from build123d import *
from build123d.topology import SkipClean

# Parameters (mm, degrees)
SKETCH2_R           = 1.65
SKETCH2_R_2         = 11.25
BOSS_EXTRUDE2_DEPTH = 2.5
SKETCH7_W           = 42.3
SKETCH7_H           = 35
BOSS_EXTRUDE5_DEPTH = 2
BOSS_EXTRUDE6_DEPTH = 2.5
FILLET2_R           = 5
FILLET3_R           = 3
SKETCH11_R          = 1.65
CUT_EXTRUDE1_DEPTH  = 2
SKETCH12_W          = 42.3
SKETCH12_H          = 35
SKETCH12_R          = 1.65
BOSS_EXTRUDE7_DEPTH = 1


with BuildPart() as part:
    # Sketch2 → Boss-Extrude2 (new, symmetric)
    with BuildSketch(Plane.XY):
        Polygon((-21.15, 16.907359313), (-16.907359313, 21.15), (16.907359313, 21.15), (21.15, 16.907359313), (21.15, -16.907359313), (21.15, -21.15), (16.907359313, -21.15), (-16.907359313, -21.15), (-21.15, -21.15), (-21.15, -16.907359313), align=None)
        with Locations((-15.5, 15.5)):
            Circle(SKETCH2_R, mode=Mode.SUBTRACT)
        Circle(SKETCH2_R_2, mode=Mode.SUBTRACT)
        with Locations((15.5, 15.5)):
            Circle(SKETCH2_R, mode=Mode.SUBTRACT)
        with Locations((15.5, -15.5)):
            Circle(SKETCH2_R, mode=Mode.SUBTRACT)
        with Locations((-15.5, -15.5)):
            Circle(SKETCH2_R, mode=Mode.SUBTRACT)
    extrude(amount=BOSS_EXTRUDE2_DEPTH, both=True)

    # Sketch7 → Boss-Extrude5 (add)
    with BuildSketch(Plane.XZ.offset(21.15)):
        with Locations((0, -15)):
            Rectangle(SKETCH7_W, SKETCH7_H)
    extrude(amount=-BOSS_EXTRUDE5_DEPTH)

    # Sketch10 → Boss-Extrude6 (add)
    with BuildSketch(Plane(origin=(21.15, 0, 0), x_dir=(0, 0, -1), z_dir=(1, 0, 0))):
        Polygon((24.130327706, -19.15), (2.5, -1), (2.5, -19.15), align=None)
    boss_extrude6 = extrude(amount=-BOSS_EXTRUDE6_DEPTH)

    # Mirror2: Boss-Extrude6 across plane
    add(boss_extrude6.mirror(Plane(origin=(0, 0, 0), x_dir=(0, 0, 1), z_dir=(1, 0, 0))))

    # Fillet2
    fillet2_edges = [part.edges().sort_by_distance(p)[0] for p in [
        (19.9, -19.15, -24.130327706),
        (19.9, -1, -2.5),
        (-19.9, -19.15, -24.130327706),
        (-19.9, -1, -2.5),
    ]]
    fillet(fillet2_edges, radius=FILLET2_R)

    # Fillet3
    # the kernel refuses this fillet: 3 mm, written as the material it takes off along each edge
    with BuildSketch(Plane(origin=(-28.221067812, -19.15, -32.5), x_dir=(0, -1, 0), z_dir=(1, 0, 0))) as fillet3_piece_1:
        with BuildLine():
            CenterArc((3, -2.828427125), FILLET3_R, 109.471220634, 70.528779366)
            Line((0, -2.828427125), (-0.06, -2.828427125))
            Line((-0.06, -2.828427125), (-0.06, 0))
            Line((-0.06, 0), (0, 0.06))
            ThreePointArc((0, 0.06), (1, 0.06), (1.98, 0.056568542))
            Line((1.98, 0.056568542), (2, 0))
        make_face()
    extrude(amount=56.442135624, mode=Mode.SUBTRACT)

    # Sketch11 → Cut-Extrude1 (cut)
    with BuildSketch(Plane(origin=(0, -19.15, 0), x_dir=(1, 0, 0), z_dir=(0, 1, 0))):
        with Locations(Location((12.5, 10, 0), (0, 0, 270))):
            Circle(SKETCH11_R)
        with Locations(Location((12.5, 25, 0), (0, 0, 270))):
            Circle(SKETCH11_R)
        with Locations(Location((-12.5, 25, 0), (0, 0, 270))):
            Circle(SKETCH11_R)
        with Locations(Location((-12.5, 10, 0), (0, 0, 270))):
            Circle(SKETCH11_R)
    extrude(amount=-CUT_EXTRUDE1_DEPTH, mode=Mode.SUBTRACT)

    # Sketch12 → Boss-Extrude7 (add)
    with SkipClean():  # the faces are left unmerged after this step: merging them gives an invalid solid
        with BuildSketch(Plane.XZ.offset(21.15)):
            with Locations((0, -15)):
                Rectangle(SKETCH12_W, SKETCH12_H)
            with Locations(Location((-12.5, -25, 0), (0, 0, 270))):
                Circle(SKETCH12_R, mode=Mode.SUBTRACT)
            with Locations(Location((-12.5, -10, 0), (0, 0, 270))):
                Circle(SKETCH12_R, mode=Mode.SUBTRACT)
            with Locations(Location((12.5, -10, 0), (0, 0, 90))):
                Circle(SKETCH12_R, mode=Mode.SUBTRACT)
            with Locations(Location((12.5, -25, 0), (0, 0, 90))):
                Circle(SKETCH12_R, mode=Mode.SUBTRACT)
        extrude(amount=BOSS_EXTRUDE7_DEPTH)
    add(part.part.scale(1), mode=Mode.REPLACE)  # the faces are merged on a copy


solid = part.part
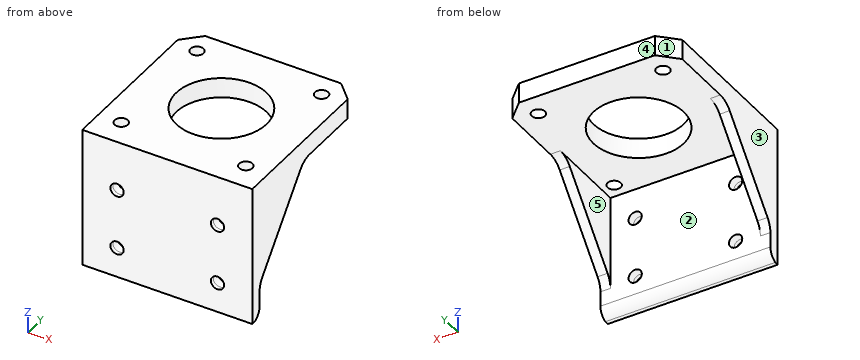
Work out the finished part from the listing and answer in its coordinate system (mm). Face numbers are marked on the shaded views. A direction names the side the tool comes from. Give positions to 0.01 mm unless a question says otherwise; leave off trailing zeros. Loops run counter-clockwise (first coordinate to the right, second up) from the corner with the lowest first, then second, coordinate; pieces in that order, holes last. Notation, with made-up numbers: (31, 18) -> (89, 18) arc R18 ccw to (89, 53) -> close; hole circle Ø3 at (-22.75, 4). An arc over 180 degrees is marked (long way). Use a Markdown table: item, result. Add a question column.
1) Consider line 1 along Z through (x, y) = (12.5, -21.65); line 2 along X through (y, z) = (-19.7, -25); line 3 along Z through (x, y) = (-12.5, -19.95). Determine where each line is inside the solid, lowest interval first.
2) The part is cut by section C-C, the plane x = 6. Determine the outline of the cut face in (y, z), plus the area to 3 significant figures.
3) The part is cut by section D-D, the plane y = 10. Determine the outline of the cut face in (x, z).
4) Each of these flat-tipped pins is pushed along its axis until it touches: P1, Ø8, axis at y = -17.5, z = -24, coming from the +X side; P2, Ø12, axis at x = -8, y = 2.5, coming from the -Z side; P3, Ø4, axis at x = -12.5, z = -25, coming from the +Y side. Where does it stop, or does it pass through?
5) Which of the six approach directions +Z, -Z, +X, -X, +Y, -Y give full straight-line access (tool end or side, diameter ignored) to the marked faces 1 and 2?
6) For a pull along X with two mould halves and no side action, classify the marked faces 3, 4 and 5 as +X half, -X half, draft (parallel to the pull), parting line (faces both ways), or undercut.
7) The part is cut by section B-B, the plane y = 15.5. Determine the outline of the cut face in (x, z).
8) The part is cut by section A-A, the plane x = -15.5. Determine the outline of the cut face in (y, z).
Reported:
| question | item | result |
|---|---|---|
| 1 | line 1 | z = -32.5 to -26.65, -23.35 to -11.65, -8.35 to 2.5 |
| 1 | line 2 | x = -21.15 to -14.15, -10.85 to 10.85, 14.15 to 21.15 |
| 1 | line 3 | z = -31.71 to -26.65, -23.35 to -11.65, -8.35 to 2.5 |
| 2 | outline | (-22.15, -32.5) -> (-21.15, -32.5) arc R3 ccw to (-19.15, -29.67) -> (-19.15, -2.5) -> (-9.52, -2.5) -> (-9.52, 2.5) -> (-22.15, 2.5) -> close; (9.52, -2.5) -> (21.15, -2.5) -> (21.15, 2.5) -> (9.52, 2.5) -> close |
| 2 | area | 210 mm^2 |
| 3 | outline | (-21.15, -2.5) -> (-5.15, -2.5) -> (-5.15, 2.5) -> (-21.15, 2.5) -> close; (5.15, -2.5) -> (21.15, -2.5) -> (21.15, 2.5) -> (5.15, 2.5) -> close |
| 4 | P1 | stops at x = 21.15 |
| 4 | P2 | stops at z = -2.5 |
| 4 | P3 | stops at y = -19.15 |
| 5 | face 1 | +Z, -Z, -X, +Y |
| 5 | face 2 | -Z, +Y |
| 6 | face 3 | -X half |
| 6 | face 4 | draft |
| 6 | face 5 | undercut |
| 7 | outline | (-21.15, -2.5) -> (-17.15, -2.5) -> (-17.15, 2.5) -> (-21.15, 2.5) -> close; (-13.85, -2.5) -> (13.85, -2.5) -> (13.85, 2.5) -> (-13.85, 2.5) -> close; (17.15, -2.5) -> (21.15, -2.5) -> (21.15, 2.5) -> (17.15, 2.5) -> close |
| 8 | outline | (-22.15, -32.5) -> (-21.15, -32.5) arc R3 ccw to (-19.15, -29.67) -> (-19.15, -2.5) -> (-17.15, -2.5) -> (-17.15, 2.5) -> (-22.15, 2.5) -> close; (-13.85, -2.5) -> (13.85, -2.5) -> (13.85, 2.5) -> (-13.85, 2.5) -> close; (17.15, -2.5) -> (21.15, -2.5) -> (21.15, 2.5) -> (17.15, 2.5) -> close |
